```python
from build123d import *

# Parameters (mm, degrees)
F0_R     = 5
F1_DEPTH = 3
F0_W     = 49
F0_H     = 49
F2_DEPTH = 1
F0_W_2   = 51
F0_H_2   = 51
F3_DEPTH = 5.5


with BuildPart() as f1:
    # F0 (on Top) → F1 (new body)
    with BuildSketch(Plane.XY):
        with Locations((20.5, 54.5)):
            Circle(F0_R)
    extrude(amount=F1_DEPTH)



with BuildPart() as f1b:
    # F0 (on Top) → F1, piece 2 (new body)
    with BuildSketch(Plane.XY):
        with Locations((37.5, 54.5)):
            Circle(F0_R)
    extrude(amount=F1_DEPTH)


with BuildPart() as f1c:
    # F0 (on Top) → F1, piece 3 (new body)
    with BuildSketch(Plane.XY):
        with Locations((54.5, 54.5)):
            Circle(F0_R)
    extrude(amount=F1_DEPTH)


with BuildPart() as f1d:
    # F0 (on Top) → F1, piece 4 (new body)
    with BuildSketch(Plane.XY):
        with Locations((54.5, 37.5)):
            Circle(F0_R)
    extrude(amount=F1_DEPTH)


with BuildPart() as f1e:
    # F0 (on Top) → F1, piece 5 (new body)
    with BuildSketch(Plane.XY):
        with Locations((37.5, 37.5)):
            Circle(F0_R)
    extrude(amount=F1_DEPTH)


with BuildPart() as f1f:
    # F0 (on Top) → F1, piece 6 (new body)
    with BuildSketch(Plane.XY):
        with Locations((20.5, 37.5)):
            Circle(F0_R)
    extrude(amount=F1_DEPTH)


with BuildPart() as f1g:
    # F0 (on Top) → F1, piece 7 (new body)
    with BuildSketch(Plane.XY):
        with Locations((20.5, 20.5)):
            Circle(F0_R)
    extrude(amount=F1_DEPTH)


with BuildPart() as f1h:
    # F0 (on Top) → F1, piece 8 (new body)
    with BuildSketch(Plane.XY):
        with Locations((37.5, 20.5)):
            Circle(F0_R)
    extrude(amount=F1_DEPTH)


with BuildPart() as f1i:
    # F0 (on Top) → F1, piece 9 (new body)
    with BuildSketch(Plane.XY):
        with Locations((54.5, 20.5)):
            Circle(F0_R)
    extrude(amount=F1_DEPTH)


with BuildPart() as f1_1:
    add(f1.part)

    add(f1b.part)  # F2 merges F1b

    add(f1c.part)  # F2 merges F1c

    add(f1d.part)  # F2 merges F1d

    add(f1e.part)  # F2 merges F1e

    add(f1f.part)  # F2 merges F1f

    add(f1g.part)  # F2 merges F1g

    add(f1h.part)  # F2 merges F1h

    add(f1i.part)  # F2 merges F1i
    # F0 (on Top) → F2 (join)
    with BuildSketch(Plane.XY):
        with Locations((37.5, 37.5)):
            Rectangle(F0_W, F0_H)
        with Locations((20.5, 20.5)):
            Circle(F0_R, mode=Mode.SUBTRACT)
        with Locations((37.5, 20.5)):
            Circle(F0_R, mode=Mode.SUBTRACT)
        with Locations((54.5, 20.5)):
            Circle(F0_R, mode=Mode.SUBTRACT)
        with Locations((20.5, 37.5)):
            Circle(F0_R, mode=Mode.SUBTRACT)
        with Locations((20.5, 54.5)):
            Circle(F0_R, mode=Mode.SUBTRACT)
        with Locations((37.5, 37.5)):
            Circle(F0_R, mode=Mode.SUBTRACT)
        with Locations((54.5, 37.5)):
            Circle(F0_R, mode=Mode.SUBTRACT)
        with Locations((37.5, 54.5)):
            Circle(F0_R, mode=Mode.SUBTRACT)
        with Locations((54.5, 54.5)):
            Circle(F0_R, mode=Mode.SUBTRACT)
    extrude(amount=F2_DEPTH)

    # F0 (on Top) → F3 (join)
    with BuildSketch(Plane.XY):
        with Locations((37.5, 37.5)):
            Rectangle(F0_W_2, F0_H_2)
        with Locations((37.5, 37.5)):
            Rectangle(F0_W, F0_H, mode=Mode.SUBTRACT)
    extrude(amount=F3_DEPTH)


solid = f1_1.part
```
Check sheet for the modelled part. Datum: model origin and axes. Units: mm. A direction names the side the tool comes from. Give positions to 0.01 mm unless a question says otherwise; leave off trailing zeros. Write each loop counter-clockwise with the first axis right and the second up, starting at its lowest first coordinate (ties: lowest second). Pieces come first, ordered by that corner, then holes. Notation, with made-up numbers: (66, 78) -> (71, 78) arc R7 cw to (71, 87) -> close; hole circle Ø3 at (-27.75, 87). An arc over 180 degrees is marked (long way). Use CSV: the item, a comma, the result in double quotes. Start each with the question number.
Q1. Tool access check on faces 1 (the flat face through (12.8, 49, 5.5)), 2 (the flat face through (13, 37, 3)). Record the directions out of +Z, -Z, +X, -X, +Y, -Y that give a thin tool (end or side, any length) a straight path to the whole face; none if there is none.
Q2. Scan lines: line 1 along Y through (x, z) = (37.5, 2.35); line 2 along Y through (x, z) = (52, 3.6); line 3 along X through (y, z) = (37, 1.45). Record each from-to range of solid material in increasing order.
Q3. Release check for a two-part mould opening along Y. For faces 3 (the flat face through (20, 38, 3)), 4 (the flat face through (37, 13, 3)), 5 (the flat face through (37, 12, 3)), 6 (the flat face through (37, 38, 0)) record: +Y half, -Y half, draft (parallel to the pull), parting line (faces both ways), or undercut.
Q4. Cross-section at B-B on x = 20.5. Enter the section's corners in (y, z).
Q5. Depth check by flat-ended pin: P1, Ø24.5, axis at x = 46, y = 42, coming from the +Z side; P2, Ø1.5, axis at x = 36.5, y = 50, coming from the -Z side; P3, Ø1, axis at x = 57, y = 26.5, coming from the +Z side. Enter the tip coordinate at first touch or a pass-through.
Q6. Cross-section at A-A on z = 2. Count the separate pieces of the cut face and the enclosed holes in it, and give its area (3 significant figures).
Q7. Cross-section at D-D on x = 50.5. Enter the section's corners in (y, z).
Q8. Cross-section at C-C on y = 48.5. Enter the section's corners in (x, z), and give its area (3 significant figures).
Working result:
1,face 1,"+Z, +X, -X, +Y, -Y"
1,face 2,"+Z"
2,line 1,"y = 12 to 13, 15.5 to 25.5, 32.5 to 42.5, 49.5 to 59.5, 62 to 63"
2,line 2,"y = 12 to 13, 62 to 63"
2,line 3,"x = 12 to 13, 15.53 to 25.47, 32.53 to 42.47, 49.53 to 59.47, 62 to 63"
3,face 3,"undercut"
3,face 4,"undercut"
3,face 5,"-Y half"
3,face 6,"draft"
4,outline,"(12, 0) -> (63, 0) -> (63, 5.5) -> (62, 5.5) -> (62, 1) -> (59.5, 1) -> (59.5, 3) -> (49.5, 3) -> (49.5, 1) -> (42.5, 1) -> (42.5, 3) -> (32.5, 3) -> (32.5, 1) -> (25.5, 1) -> (25.5, 3) -> (15.5, 3) -> (15.5, 1) -> (13, 1) -> (13, 5.5) -> (12, 5.5) -> close"
5,P1,"stops at z = 3"
5,P2,"stops at z = 0"
5,P3,"stops at z = 1"
6,separate pieces,"10"
6,enclosed holes,"1"
6,area,"907 mm^2"
7,outline,"(12, 0) -> (63, 0) -> (63, 5.5) -> (62, 5.5) -> (62, 1) -> (57.5, 1) -> (57.5, 3) -> (51.5, 3) -> (51.5, 1) -> (40.5, 1) -> (40.5, 3) -> (34.5, 3) -> (34.5, 1) -> (23.5, 1) -> (23.5, 3) -> (17.5, 3) -> (17.5, 1) -> (13, 1) -> (13, 5.5) -> (12, 5.5) -> close"
8,outline,"(12, 0) -> (63, 0) -> (63, 5.5) -> (62, 5.5) -> (62, 1) -> (13, 1) -> (13, 5.5) -> (12, 5.5) -> close"
8,area,"60.0 mm^2"
